CAD build for the part. Positions are in the model's coordinates, mm. Face numbers are marked on the shaded views. Coordinates: 2 decimals unless noted, no trailing zeros. Loops run counter-clockwise (first coordinate to the right, second up) from the corner with the lowest first, then second, coordinate; pieces in that order, holes last. Notation, with made-up numbers: (86.5, 75) -> (120.5, 75) arc R22 cw to (120.5, 107) -> close; hole circle Ø5 at (42.5, -14). An arc over 180 degrees is marked (long way). Write item = value, one per line. Start each with the question number.
(1) Band-saw the part on C-C (z = 20.4). Write the cut outline in (x, y).
(2) Band-saw the part on D-D (x = -24.75). Write the cut outline in (y, z), and give its area (3 significant figures).
(3) Flat gauge pin, fed straight in: P1, Ø1, axis at y = 49.5, z = 21, coming from the -X side. Where does the tip first touch, or does it go through?
(4) Band-saw the part on A-A (y = 53.1). Write the cut outline in (x, z).
(5) Drill centre lines: line 1 (Y direction, x = -29.1, z = 20.4); line 2 (Y direction, x = -28.5, z = 19.65); line 3 (X direction, y = 54.5, z = 20.25). Where is each one in solid material? Low to high. Write a range as from..to.
(6) Band-saw the part on B-B (x = -29.1). Write the cut outline in (y, z), and give its area (3 significant figures).
(7) Pull direction Y, two halves, no side cores. Call the marked faces 1, 2 and 3: +Y half, -Y half, draft (parallel to the pull), parting line (faces both ways), or undercut.
```python
from build123d import *

# Parameters (mm, degrees)
CYLINDER013_R     = 1.8
CYLINDER013_DEPTH = 5
CYLINDER012_R     = 5.5
CYLINDER012_DEPTH = 2


with BuildPart() as obj1:
    # Cylinder013 → Cylinder013 (new body)
    with BuildSketch(Plane(origin=(-29.1, 53.1, 24.6), x_dir=(1, 0, 0), z_dir=(0, 0, 1))):
        Circle(CYLINDER013_R)
    extrude(amount=CYLINDER013_DEPTH)


with BuildPart() as arandela_2mm:
    # Cylinder012 → Cylinder012 (new body)
    with BuildSketch(Plane(origin=(-29.1, 53.1, 25.2), x_dir=(1, 0, 0), z_dir=(0, 0, 1))):
        Circle(CYLINDER012_R)
    extrude(amount=CYLINDER012_DEPTH)

    # Cut006: cut obj1
    add(obj1.part, mode=Mode.SUBTRACT)


with BuildPart() as arandela_2mm_1:
    # Cut006 placement: moved
    add(arandela_2mm.part.moved(Location((0, 0, -5.7))))


solid = arandela_2mm_1.part
```
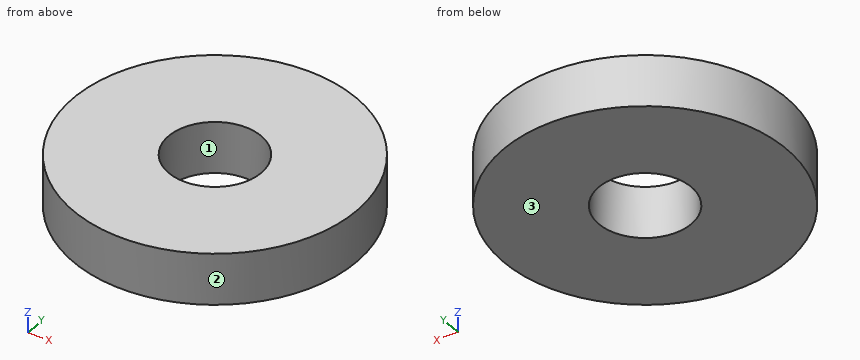
Findings below:
q1.outline = circle Ø11 at (-29.1, 53.1); hole circle Ø3.6 at (-29.1, 53.1)
q2.outline = (49.73, 19.5) -> (56.47, 19.5) -> (56.47, 21.5) -> (49.73, 21.5) -> close
q2.area = 13.5 mm²
q3.P1 = -33.64
q4.outline = (-34.6, 19.5) -> (-30.9, 19.5) -> (-30.9, 21.5) -> (-34.6, 21.5) -> close; (-27.3, 19.5) -> (-23.6, 19.5) -> (-23.6, 21.5) -> (-27.3, 21.5) -> close
q5.line_1 = 47.6..51.3, 54.9..58.6
q5.line_2 = 47.63..51.4, 54.8..58.57
q5.line_3 = -34.42..-30.23, -27.97..-23.78
q6.outline = (47.6, 19.5) -> (51.3, 19.5) -> (51.3, 21.5) -> (47.6, 21.5) -> close; (54.9, 19.5) -> (58.6, 19.5) -> (58.6, 21.5) -> (54.9, 21.5) -> close
q6.area = 14.8 mm²
q7.face_1 = undercut
q7.face_2 = parting line
q7.face_3 = draft
